Can you work these out from the model? Positions are in its coordinate system, mm. Face numbers are marked on the shaded views. A direction names the side the tool comes from. Coordinates: 2 decimals unless noted, no trailing zeros. Loops run counter-clockwise (first coordinate to the right, second up) from the corner with the lowest first, then second, coordinate; pieces in that order, holes last.
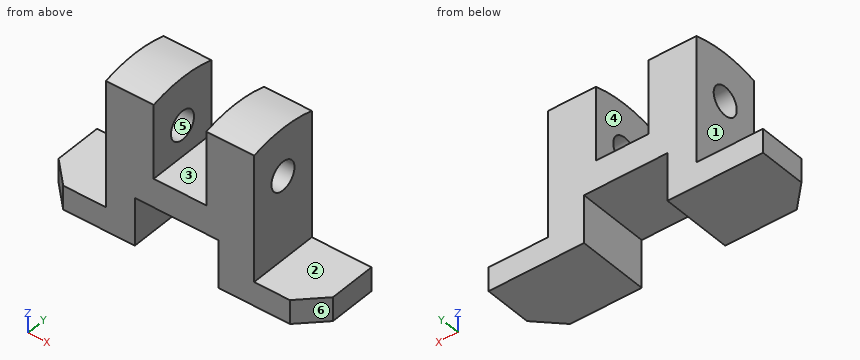
Autodesk Fusion 360 part; units mm, degrees
sketch "Sketch1" plane through (0, 0, 0) normal (0, 1, 0) x (1, 0, 0)
  line L0 (-20, -5) -> (-20, 5)
  line L1 (-20, 5) -> (20, 5)
  line L2 (20, 5) -> (20, -15)
  line L3 (20, -15) -> (55, -15)
  line L4 (55, -15) -> (55, 5)
  line L5 (55, 5) -> (85, 5)
  line L6 (85, 5) -> (95, 5)
  line L7 (95, 5) -> (95, -5)
  line L8 (95, -5) -> (70, -5)
  line L9 (70, -5) -> (70, -60)
  line L10 (70, -60) -> (50, -60)
  line L11 (50, -60) -> (50, -27)
  line L12 (50, -27) -> (27.9096, -27)
  line L13 (27.9096, -27) -> (27.9096, -60)
  line L14 (27.9096, -60) -> (7.9096, -60)
  line L15 (7.9096, -60) -> (7.9096, -5)
  line L16 (7.9096, -5) -> (-20, -5)
  dimension "d2" = 20
extrude "Extrude1" add sketch "Sketch1" along normal mid plane 30
chamfer "Chamfer1" distance 10 angle 45 2 edges at (-20, -15, 0) (95, -15, 0)
sketch "Sketch2" plane through (70, 0, 0) normal (1, 0, 0) x (0, 1, 0)
  line L0 (-15, 5) -> (15, 5)
  line L1 (15, 5) -> (15, 60)
  line L2 (15, 60) -> (-15, 60)
  line L3 (-15, 60) -> (-15, 5)
  point P0 (0, 40)
hole "Hole1" at (70, 0, 40) direction (-1, 0, 0) diameter 12 depth 65 tip angle 118
sketch "Sketch4" plane through (7.9096, 0, 0) normal (-1, 0, 0) x (0, -1, 0)
  circle A0 centre (0, 40) radius 6
  line L0 (15, 60) -> (-15, 60)
  line L1 (-15, 60) -> (-15, 5)
  line L2 (-15, 5) -> (15, 5)
  line L3 (15, 5) -> (15, 60)
  circle A1 centre (0, 5) radius 55
extrude "Extrude2" cut sketch "Sketch4" against normal blind 12311 contours L0 L3 A1 | L0 L1 A1
Item 1: Suppose I cut it at D-D, the plane y = 9.5. Please give me the cut outline in (x, z).
Results are:
outline: (-20, -5) - (20, -5) - (20, 15) - (55, 15) - (55, -5) - (95, -5) - (95, 5) - (70, 5) - (70, 59.17) - (50, 59.17) - (50, 27) - (27.91, 27) - (27.91, 59.17) - (7.91, 59.17) - (7.91, 5) - (-20, 5) - close
Item 2: Suppose I cut it at A-A, the plane y = 0. Please give me the cut outline in (x, z).
Results are:
outline: (-20, -5) - (20, -5) - (20, 15) - (55, 15) - (55, -5) - (95, -5) - (95, 5) - (70, 5) - (70, 34) - (50, 34) - (50, 27) - (27.91, 27) - (27.91, 34) - (7.91, 34) - (7.91, 5) - (-20, 5) - close; (7.91, 46) - (27.91, 46) - (27.91, 60) - (7.91, 60) - close; (50, 46) - (70, 46) - (70, 60) - (50, 60) - close
Item 3: I'm going to push flat-ended pins straight in: P1, Ø8, axis at y = 9, z = 43.5, coming from the -X side; P2, Ø14, axis at x = -8.5, y = 5, coming from the +Z side; P3, Ø5, axis at x = 45, y = -1.5, coming from the -Z side; P4, Ø7, axis at y = 0, z = 40, coming from the -X side. Where does each tip first touch, or does it pass through?
Results are:
P1: stops at x = 7.91
P2: stops at z = 5
P3: stops at z = 15
P4: passes through
Item 4: I need wall thicknesses on line 1 along Z through (x, y) = (18, 0); line 2 along Y through (x, z) = (21, 40); line 3 along X through (y, z) = (7, 30). Which ranges of each line are inside material? Lowest first, please.
Results are:
line 1: z = -5 to 34, 46 to 60
line 2: y = -15 to -6, 6 to 15
line 3: x = 7.91 to 27.91, 50 to 70
Item 5: We'd pull the mould along X, two halves only. Please class the marked faces 4, 5 and 6: +X half, -X half, draft (parallel to the pull), parting line (faces both ways), or undercut.
Results are:
face 4: undercut
face 5: draft
face 6: +X half
Item 6: Suppose I cut it at B-B, the plane z = 40. Please give me the cut outline in (x, y).
Results are:
outline: (7.91, -15) - (27.91, -15) - (27.91, -6) - (7.91, -6) - close; (7.91, 6) - (27.91, 6) - (27.91, 15) - (7.91, 15) - close; (50, -15) - (70, -15) - (70, -6) - (50, -6) - close; (50, 6) - (70, 6) - (70, 15) - (50, 15) - close
Item 7: On a 3-axis mill with a long thin cutter (end or side, diameter ignored), from which of +Z, -Z, +X, -X, +Y, -Y can I reach the whole of each face in a straight line? I mean the marked faces 1, 2 and 3. Say none if no direction works.
Results are:
face 1: +Z, -X, +Y, -Y
face 2: +Z, +X, +Y, -Y
face 3: +Z, +Y, -Y
Item 8: Suppose I cut it at C-C, the plane x = 16. Please give me the cut outline in (y, z), plus the area to 3 significant figures.
Results are:
outline: (-15, -5) - (15, -5) - (15, 57.92) arc R55 ccw to (-15, 57.92) - close; hole circle Ø12 at (0, 40)
area: 1,820 mm2
